Can you work these out from the model? Positions are in its coordinate system, mm. Face numbers are marked on the shaded views. A direction names the side the tool comes from. Coordinates: 2 decimals unless noted, no trailing zeros. Loops run counter-clockwise (first coordinate to the right, second up) from the corner with the lowest first, then second, coordinate; pieces in that order, holes last. Notation, with made-up numbers: (33.25, 71.5) -> (80.25, 71.5) arc R15 cw to (80.25, 88.5) -> close; hole circle Ø1 at (26, -23.75). An arc over 180 degrees is marked (long way). Put each result on its own line as item: value. Start each with the question number.
Item 1: We'd pull the mould along Y, two halves only. Please class the marked faces 1, 2, 3 and 4: pulls with the +Y half, pulls with the -Y half, needs draft (parallel to the pull), parting line crosses it, or undercut.
Item 2: If we section it at D-D on x = 0: Please give me the cut outline in (y, z).
Item 3: If we section it at B-B on x = 101.6: Please give me the cut outline in (y, z), plus the area to 3 significant figures.
Item 4: Please list where these lines run through material, in increasing order: L1, parallel to Y at x = 0, z = 71.5; L2, parallel to Y at x = 0, z = 16.5; L3, parallel to X at y = -8, z = 32.5. Write a range as from..to.
Item 5: For the marked faces 5, 6, 7, 8 and 9, which set-ups out of +Z, -Z, +X, -X, +Y, -Y let a thin tool reach every point of the face, with its end or its side?
Item 6: If we section it at C-C on z = 47: Please give me the cut outline in (x, y) (3 decimals), plus the area to 3 significant figures.
Item 7: If we section it at A-A on y = 0: Please give me the cut outline in (x, z), plus the area to 3 significant figures.
Item 8: Will these pins go through, and if not, where does the flat tip stop? P1, Ø10, axis at x = 7.5, z = 43.5, coming from the +Y side; P2, Ø6, axis at x = -11.5, y = -35.5, coming from the +Z side; P3, Ø10, axis at y = -14, z = 14.5, coming from the -X side; P4, Ø1.5, axis at x = 12, y = 38.5, coming from the +Z side.
```python
from build123d import *

# Parameters (mm, degrees)
F0_R     = 21.971
F1_DEPTH = 38.1
F2_DEPTH = 63.5
F5_DEPTH = 25.4
F6_R     = 50.6512427991
F6_R_2   = 40.8739745441
F7_DEPTH = 25.4


with BuildPart() as f1:
    # F0 (on Top) → F1 (new body)
    with BuildSketch(Plane.XY):
        with BuildLine():
            ThreePointArc((8.89, -50.0160764155), (38.9374626806, -32.6268907498), (50.8, 0))
            ThreePointArc((50.8, 0), (38.9374626806, 32.6268907498), (8.89, 50.0160764155))
            ThreePointArc((8.89, 50.0160764155), (-50.8, 0), (8.89, -50.0160764155))
        make_face()
        with BuildLine():
            ThreePointArc((-19.7989700742, 9.525), (0, 21.971), (19.7989700742, 9.525))
            Line((19.7989700742, 9.525), (31.75, 9.525))
            Line((31.75, 9.525), (31.75, -9.525))
            Line((31.75, -9.525), (19.7989700742, -9.525))
            ThreePointArc((19.7989700742, -9.525), (0, -21.971), (-19.7989700742, -9.525))
            Line((-19.7989700742, -9.525), (-31.75, -9.525))
            Line((-31.75, -9.525), (-31.75, 9.525))
            Line((-31.75, 9.525), (-19.7989700742, 9.525))
        make_face(mode=Mode.SUBTRACT)
        with BuildLine():
            ThreePointArc((8.89, 50.0160764155), (38.9374626806, 32.6268907498), (50.8, 0))
            ThreePointArc((50.8, 0), (38.9374626806, -32.6268907498), (8.89, -50.0160764155))
            Line((8.89, -50.0160764155), (107.3785, -32.5104496701))
            ThreePointArc((107.3785, -32.5104496701), (68.58, 0), (107.3785, 32.5104496701))
            Line((107.3785, 32.5104496701), (8.89, 50.0160764155))
        make_face()
        with BuildLine():
            ThreePointArc((134.62, 0), (126.9093507424, 21.2074789874), (107.3785, 32.5104496701))
            ThreePointArc((107.3785, 32.5104496701), (68.58, 0), (107.3785, -32.5104496701))
            ThreePointArc((107.3785, -32.5104496701), (126.9093507424, -21.2074789874), (134.62, 0))
        make_face()
        with Locations((101.6, 0)):
            Circle(F0_R, mode=Mode.SUBTRACT)
        with BuildLine():
            ThreePointArc((-19.7989700742, -9.525), (-21.971, 0), (-19.7989700742, 9.525))
            Line((-19.7989700742, 9.525), (-31.75, 9.525))
            Line((-31.75, 9.525), (-31.75, -9.525))
            Line((-31.75, -9.525), (-19.7989700742, -9.525))
        make_face()
    extrude(amount=F1_DEPTH)

    # F0 (on Top) → F2 (join)
    with BuildSketch(Plane.XY):
        with BuildLine():
            ThreePointArc((8.89, -50.0160764155), (38.9374626806, -32.6268907498), (50.8, 0))
            ThreePointArc((50.8, 0), (38.9374626806, 32.6268907498), (8.89, 50.0160764155))
            ThreePointArc((8.89, 50.0160764155), (-50.8, 0), (8.89, -50.0160764155))
        make_face()
        with BuildLine():
            ThreePointArc((-19.7989700742, 9.525), (0, 21.971), (19.7989700742, 9.525))
            Line((19.7989700742, 9.525), (31.75, 9.525))
            Line((31.75, 9.525), (31.75, -9.525))
            Line((31.75, -9.525), (19.7989700742, -9.525))
            ThreePointArc((19.7989700742, -9.525), (0, -21.971), (-19.7989700742, -9.525))
            Line((-19.7989700742, -9.525), (-31.75, -9.525))
            Line((-31.75, -9.525), (-31.75, 9.525))
            Line((-31.75, 9.525), (-19.7989700742, 9.525))
        make_face(mode=Mode.SUBTRACT)
        with BuildLine():
            ThreePointArc((-19.7989700742, -9.525), (-21.971, 0), (-19.7989700742, 9.525))
            Line((-19.7989700742, 9.525), (-31.75, 9.525))
            Line((-31.75, 9.525), (-31.75, -9.525))
            Line((-31.75, -9.525), (-19.7989700742, -9.525))
        make_face()
    extrude(amount=F2_DEPTH)

    # F4 (on face) → F5 (join)
    with BuildSketch(Plane(origin=(8.89, -50.0160764155, 0), x_dir=(0.9845684334, 0.175, 0), z_dir=(0.175, -0.9845684334, 0))):
        Polygon((64.2408422213, 8.1636081304), (70.6394698458, 18.9178303739), (67.0485100533, 25.3305059427), (59.4336241402, 20.8529178065), (59.3616303693, 29.9041031382), (52.0126105242, 30.0005785183), (45.6139828997, 19.2463562748), (51.7280987483, 8.3278710809), align=None)
        Polygon((59.4336241402, 20.8529178065), (67.0485100533, 25.3305059427), (64.5253539973, 29.8363155678), (59.3616303693, 29.9041031382), align=None)
        Polygon((64.5253539973, 29.8363155678), (67.0485100533, 25.3305059427), (74.8510695994, 29.9184470431), (59.2913682522, 38.7375818539), (59.3616303693, 29.9041031382), align=None)
    extrude(amount=F5_DEPTH)

    # F6 (on face) → F7 (join)
    with BuildSketch(Plane.XY.offset(63.5)):
        Circle(F6_R)
        Circle(F6_R_2, mode=Mode.SUBTRACT)
    extrude(amount=F7_DEPTH)


solid = f1.part
```
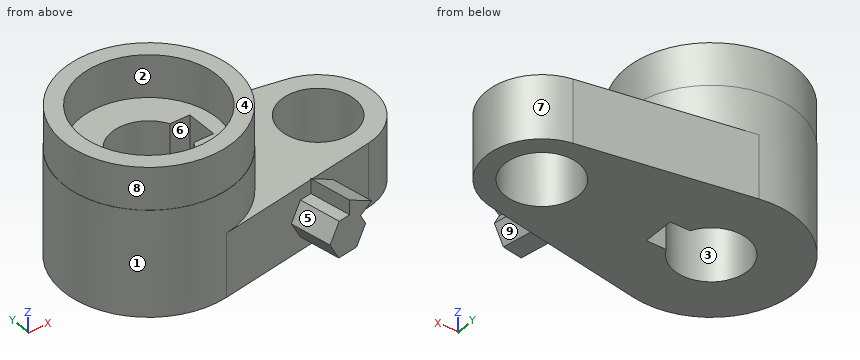
Solutions:
1. face 1: parting line crosses it
1. face 2: undercut
1. face 3: undercut
1. face 4: needs draft
2. outline: (-50.8, 0) -> (-21.97, 0) -> (-21.97, 63.5) -> (-40.87, 63.5) -> (-40.87, 88.9) -> (-50.65, 88.9) -> (-50.65, 63.5) -> (-50.8, 63.5) -> close; (21.97, 0) -> (50.8, 0) -> (50.8, 63.5) -> (50.65, 63.5) -> (50.65, 88.9) -> (40.87, 88.9) -> (40.87, 63.5) -> (21.97, 63.5) -> close
3. outline: (-33.54, 0) -> (-21.97, 0) -> (-21.97, 38.1) -> (-33.54, 38.1) -> close; (21.97, 0) -> (33.54, 0) -> (33.54, 38.1) -> (21.97, 38.1) -> close
3. area: 881 mm^2
4. L1: -50.65..-40.87, 40.87..50.65
4. L2: -50.8..-21.97, 21.97..50.8
4. L3: -50.17..-20.46, 31.75..81.14, 122.06..133.64
5. face 5: +Z, -Y
5. face 6: +Z, -Z
5. face 7: +Z, -Z, +X
5. face 8: +Z
5. face 9: -Z, +X
6. outline: circle Ø101.6 at (0, 0); hole (19.799, -9.525) -> (31.75, -9.525) -> (31.75, 9.525) -> (19.799, 9.525) arc R21.971 ccw (long way) to start
6. area: 6,390 mm^2
7. outline: (-50.8, 0) -> (-21.97, 0) -> (-21.97, 63.5) -> (-40.87, 63.5) -> (-40.87, 88.9) -> (-50.65, 88.9) -> (-50.65, 63.5) -> (-50.8, 63.5) -> close; (31.75, 0) -> (79.63, 0) -> (79.63, 38.1) -> (50.8, 38.1) -> (50.8, 63.5) -> (50.65, 63.5) -> (50.65, 88.9) -> (40.87, 88.9) -> (40.87, 63.5) -> (31.75, 63.5) -> close; (123.57, 0) -> (134.62, 0) -> (134.62, 38.1) -> (123.57, 38.1) -> close
7. area: 5,060 mm^2
8. P1: y = 50.74
8. P2: z = 63.5
8. P3: x = -50
8. P4: z = 88.9
